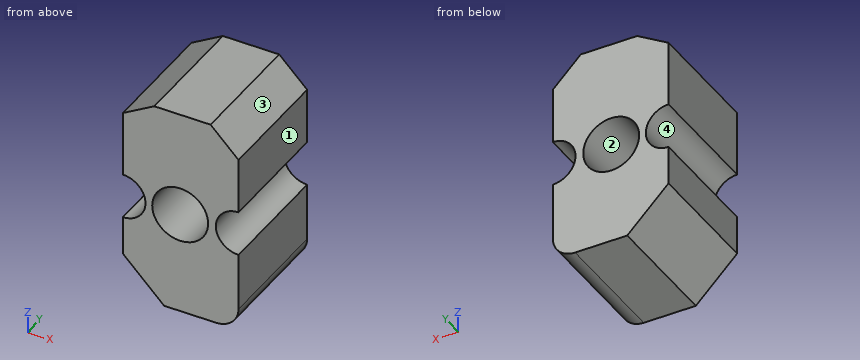
Autodesk Inventor part; units mm, degrees
ref_plane "YZ Plane" through (0, 0, 0) normal (1, 0, 0) x (0, 1, 0)
ref_plane "XZ Plane" through (0, 0, 0) normal (0, 1, 0) x (-1, 0, 0)
ref_plane "XY Plane" through (0, 0, 0) normal (0, 0, 1) x (1, 0, 0)
sketch "Sketch1" plane through (0, 0, 0) normal (0, 0, 1) x (1, 0, 0)
  point P0 (0, 0)
sketch "Sketch2" plane through (0, 0, 0) normal (0, 1, 0) x (-1, 0, 0)
  line L0 (18.3793, 32.1145) -> (-18.6207, 32.1145)
  line L1 (-18.6207, 32.1145) -> (-18.6207, -28.8855)
  line L2 (-18.6207, -28.8855) -> (18.3793, -28.8855)
  line L3 (18.3793, -28.8855) -> (18.3793, 32.1145)
  line L4 (-18.6207, 32.1145) -> (-18.6207, 28.0145)
  line L5 (-18.6207, 28.0145) -> (-14.5207, 28.0145)
  line L6 (-14.5207, 28.0145) -> (-7.6207, 28.0145)
  line L7 (-7.6207, 28.0145) -> (6.2793, 28.0145)
  line L8 (6.2793, 28.0145) -> (14.2793, 28.0145) construction
  line L9 (14.0338, 32.3374) -> (14.0338, 23.5374)
  line L10 (6.2793, 28.0145) -> (14.0338, 23.5374)
  line L11 (14.0338, 23.5374) -> (14.0338, 7.3145)
  arc A0 (14.0338, 7.3145) -> (14.0338, -3.8855) centre (14.0338, 1.7145) ccw
  line L12 (14.0338, -3.8855) -> (14.0338, -13.4855)
  arc A1 (-14.5207, -3.8855) -> (-14.5207, 7.3145) centre (-14.5207, 1.7145) ccw
  line L13 (-14.5207, -3.8855) -> (-14.5207, -18.1855)
  line L14 (-7.6207, 28.0145) -> (-14.5207, 21.1145)
  line L15 (-14.5207, 32.1145) -> (-14.5207, 28.0145)
  line L16 (-14.5207, 21.1145) -> (-14.5207, 7.3145)
  line L17 (-14.5207, -18.1855) -> (-14.5207, -23.6855) construction
  line L18 (-14.5207, -23.6855) -> (3.8338, -23.6855)
  line L19 (14.0338, -13.4855) -> (3.8338, -23.6855)
  line L20 (-1.3662, -28.8855) -> (-1.8697, -29.389)
  arc A2 (-14.5207, -18.1855) -> (-9.0207, -23.6855) centre (-9.0207, -18.1855) ccw
  line L21 (14.0338, 1.7145) -> (-14.5207, 1.7145)
  circle A3 centre (-0.1207, 1.7145) radius 6.9
  point P0 (0, 0)
  dimension "d2" = 37
  dimension "d3" = 61
  dimension "d4" = 4.1
  dimension "d5" = 4.1
  dimension "d6" = 6.9
  dimension "d7" = 13.9
  dimension "d9" = 8.8
  dimension "d10" = 30
  dimension "d12" = 30.4
  dimension "d13" = 24.8
  dimension "d14" = 45.6
  dimension "d16" = 24.8
  dimension "d17" = 30.4
  dimension "d20" = 50.3
  dimension "d21" = 45
  dimension "d22" = 5.5
  dimension "d24" = 5.5
  dimension "d25" = 5.5
  dimension "d26" = 18.5
  dimension "d27" = 13.8
extrude "Extrusion1" add sketch "Sketch2" against normal blind 30 contours L11 A0 L21 A3 A1 L16 L14 L7 L10 | A0 L12 L19 L18 A2 L13 A1 L21 A3
sketch "Sketch3" plane through (0, 0, 0) normal (0, 1, 0) x (1, 0, 0)
  line L0 (7.6207, -28.0145) -> (-6.2793, -28.0145)
  line L1 (7.6207, -28.0145) -> (14.5207, -21.1145)
  line L2 (14.5207, -21.1145) -> (14.5207, -7.3145)
  arc A0 (14.5207, 3.8855) -> (14.5207, -7.3145) centre (14.5207, -1.7145) ccw
  line L3 (14.5207, 3.8855) -> (14.5207, 18.1855)
  arc A1 (14.5207, 18.1855) -> (9.0207, 23.6855) centre (9.0207, 18.1855) ccw
  line L4 (9.0207, 23.6855) -> (-3.8338, 23.6855)
  line L5 (-3.8338, 23.6855) -> (-14.0338, 13.4855)
  line L6 (-14.0338, 13.4855) -> (-14.0338, 3.8855)
  arc A2 (-14.0338, -7.3145) -> (-14.0338, 3.8855) centre (-14.0338, -1.7145) ccw
  line L7 (-14.0338, -23.5374) -> (-14.0338, -7.3145)
  line L8 (-14.0338, -23.5374) -> (-6.2793, -28.0145)
  circle A3 centre (0.1207, -1.7145) radius 6.9
  point P0 (0, 0)
  point P1 (14.5207, -28.0145)
Here's how the part is built. I have some questions about the finished solid (model axes, mm). Face numbers are marked on the shaded views. Give positions to 0.01 mm unless a question says otherwise; leave off trailing zeros. Write each loop counter-clockwise with the first axis right and the second up, starting at its lowest first coordinate (ties: lowest second). Pieces come first, ordered by that corner, then holes.
(1) Will these pins go through, and if not, where does the flat tip stop? pin 1 (1.5 mm diameter, centred on x = 11.5, y = -14, fed in from +Z); pin 2 (12 mm diameter, centred on x = -4.5, y = -8, fed in from -Z); pin 3 (1 mm diameter, centred on x = 11.5, y = -22.5, fed in from +Z).
Output values:
pin 1: stops at z = 24.89
pin 2: stops at z = -23.69
pin 3: stops at z = 24.64
(2) Imagine slicing it at B-B, the plane x = 10.75. Write out the boundary of the cut face in (y, z).
Output values:
outline: (-30, -23.41) - (0, -23.41) - (0, -2.43) - (-30, -2.43) - close; (-30, 5.85) - (0, 5.85) - (0, 24.89) - (-30, 24.89) - close
(3) If I drill on L1, parallel to Z at x = 3.75, y = -21; L2, parallel to Z at x = -2.25, y = -24.5; L3, parallel to X at y = -15.75, z = 5.5, over which ranges is the centre line in solid material (lowest first)?
Output values:
L1: z = -23.69 to -4.15, 7.58 to 28.01
L2: z = -23.69 to -4.77, 8.19 to 28.01
L3: x = -9.91 to -5.65, 5.89 to 10.39
(4) Thinking about a two-plate mould opening in Z: for the marked faces 1, 2, 3 and 4, which applies, pulls with the +Z half, pulls with the -Z half, needs draft (parallel to the pull), parting line crosses it, or undercut?
Output values:
face 1: needs draft
face 2: undercut
face 3: pulls with the +Z half
face 4: undercut
(5) Imagine slicing it at C-C, the plane y = -9.5. Write out the boundary of the cut face in (x, z), and give its area (3 significant figures).
Output values:
outline: (-14.03, -13.49) - (-3.83, -23.69) - (9.02, -23.69) arc R5.5 ccw to (14.52, -18.19) - (14.52, -3.89) arc R5.6 cw to (14.52, 7.31) - (14.52, 21.11) - (7.62, 28.01) - (-6.28, 28.01) - (-14.03, 23.54) - (-14.03, 7.31) arc R5.6 cw to (-14.03, -3.89) - close; hole circle Ø13.8 at (0.12, 1.71)
area: 1,130 mm2
(6) Imagine slicing it at D-D, the plane z = -19. Write out the boundary of the cut face in (x, y).
Output values:
outline: (-8.52, -30) - (14.46, -30) - (14.46, 0) - (-8.52, 0) - close
(7) Imagine slicing it at A-A, the plane z = -3. Write out the boundary of the cut face in (x, y), and give its area (3 significant figures).
Output values:
outline: (-11.01, -30) - (-4.92, -30) - (-4.92, 0) - (-11.01, 0) - close; (5.16, -30) - (11.5, -30) - (11.5, 0) - (5.16, 0) - close
area: 373 mm2
